```python
from build123d import *

# Parameters (mm, degrees)
EXTRUDE_1_DEPTH     = 10
SKETCH_2_R          = 16
SKETCH_2_R_2        = 11
CUT_EXTRUDE_1_DEPTH = 10


with BuildPart() as part:
    # 草图1 → 凸台-拉伸1 (new body)
    with BuildSketch(Plane.XY):
        with BuildLine():
            ThreePointArc((9.384103149, 51.455229093), (0, 58), (-9.384103149, 51.455229093))
            ThreePointArc((-9.384103149, 51.455229093), (-17.720006387, 42.779879746), (-29.748778447, 43.019904391))
            ThreePointArc((-29.748778447, 43.019904391), (-41.012193309, 41.012193309), (-43.019904391, 29.748778447))
            ThreePointArc((-43.019904391, 29.748778447), (-42.779879746, 17.720006387), (-51.455229093, 9.384103149))
            ThreePointArc((-51.455229093, 9.384103149), (-58, 0), (-51.455229093, -9.384103149))
            ThreePointArc((-51.455229093, -9.384103149), (-42.779879746, -17.720006387), (-43.019904391, -29.748778447))
            ThreePointArc((-43.019904391, -29.748778447), (-41.012193309, -41.012193309), (-29.748778447, -43.019904391))
            ThreePointArc((-29.748778447, -43.019904391), (-17.720006387, -42.779879746), (-9.384103149, -51.455229093))
            ThreePointArc((-9.384103149, -51.455229093), (0, -58), (9.384103149, -51.455229093))
            ThreePointArc((9.384103149, -51.455229093), (17.720006387, -42.779879746), (29.748778447, -43.019904391))
            ThreePointArc((29.748778447, -43.019904391), (41.012193309, -41.012193309), (43.019904391, -29.748778447))
            ThreePointArc((43.019904391, -29.748778447), (42.779879746, -17.720006387), (51.455229093, -9.384103149))
            ThreePointArc((51.455229093, -9.384103149), (58, 0), (51.455229093, 9.384103149))
            ThreePointArc((51.455229093, 9.384103149), (42.779879746, 17.720006387), (43.019904391, 29.748778447))
            ThreePointArc((43.019904391, 29.748778447), (41.012193309, 41.012193309), (29.748778447, 43.019904391))
            ThreePointArc((29.748778447, 43.019904391), (17.720006387, 42.779879746), (9.384103149, 51.455229093))
        make_face()
    extrude(amount=EXTRUDE_1_DEPTH)

    # 草图2 → 切除-拉伸1 (cut)
    with BuildSketch(Plane.XY.offset(10)):
        Circle(SKETCH_2_R)
        with Locations((0, 32)):
            Circle(SKETCH_2_R_2)
        with Locations((32, 0)):
            Circle(SKETCH_2_R_2)
        with Locations((0, -32)):
            Circle(SKETCH_2_R_2)
        with Locations((-32, 0)):
            Circle(SKETCH_2_R_2)
    extrude(amount=-CUT_EXTRUDE_1_DEPTH, mode=Mode.SUBTRACT)


solid = part.part
```
Input: part model. Units: mm. Frame: model coordinates. Give positions to 0.01 mm unless a question says otherwise; leave off trailing zeros. Loops run counter-clockwise (first coordinate to the right, second up) from the corner with the lowest first, then second, coordinate; pieces in that order, holes last. Notation, with made-up numbers: M 52.5,-21 L 99.5,-21 A37 ccw 99.5,15 Z; hole C 42,5 d9. An arc over 180 degrees is marked long. Answer as CSV lines item,"result". Start each with the question number.
1. Line query: L1, parallel to X at y = -9, z = 5; L2, parallel to Y at x = 36, z = 8.5; L3, parallel to Y at x = 32, z = 3.75. Output: solid intervals per line, ascending.
2. Section A-A on y = 0. Return loops of the section in (x, z), plus the area to 3 significant figures.
3. Section C-C on y = -32. Return loops of the section in (x, z).
4. Pin query (flat end, axial travel): P1, Ø1.5, axis at x = 40, z = 2, coming from the +Y side; P2, Ø5, axis at x = 3.5, z = 5.5, coming from the +Y side; P3, Ø5, axis at y = 40.5, z = 7.5, coming from the +X side. Return the tip coordinate at first contact, or that it passes through.
5. Pull-direction query (X, two-part tool) for faces 1 (the face through (0, -58, 5)), 2 (the face through (42.161, -4.213, 5.07)), 3 (the face through (42.714, -17.881, 4.93)); classes: released by +X, released by -X, zero draft, split by the parting line, or undercut.
Computed values:
1,L1,"x = -52.36 to -38.32, -25.68 to -13.23, 13.23 to 25.68, 38.32 to 52.36"
1,L2,"y = -43.73 to -10.25, 10.25 to 43.73"
1,L3,"y = -43.75 to -11, 11 to 43.75"
2,outline,"M -58,0 L -43,0 L -43,10 L -58,10 Z; M -21,0 L -16,0 L -16,10 L -21,10 Z; M 16,0 L 21,0 L 21,10 L 16,10 Z; M 43,0 L 58,0 L 58,10 L 43,10 Z"
2,area,"400 mm²"
3,outline,"M -43.75,0 L -11,0 L -11,10 L -43.75,10 Z; M 11,0 L 43.75,0 L 43.75,10 L 11,10 Z"
4,P1,"stops at y = 42.42"
4,P2,"stops at y = 57.95"
4,P3,"stops at x = 43.08"
5,face 1,"split by the parting line"
5,face 2,"undercut"
5,face 3,"released by +X"
